from build123d import *

# Parameters (mm, degrees)
EXTRUDE_1_DEPTH        = 4
SKETCH_2_R             = 1.525
CUT_EXTRUDE_1_DEPTH    = 5
FILLET_1_R             = 3
SKETCH_3_R             = 1.8
CUT_EXTRUDE_5_DEPTH    = 5
CUT_EXTRUDE_3_DEPTH    = 5
FILLET_2_R             = 1.5
FILLET_2_OF_MIRROR_1_R = 1.5
SKETCH_5_R             = 9
CUT_EXTRUDE_4_DEPTH    = 5


with BuildPart() as part:
    # 草图1 → 凸台-拉伸1 (new body)
    with BuildSketch(Plane(origin=(0, 0, 0), x_dir=(1, 0, 0), z_dir=(0, 1, 0))):
        with BuildLine():
            Line((-20, 18), (-20, -18))
            Line((-20, -18), (20, -18))
            ThreePointArc((20, -18), (2, 0), (20, 18))
            Line((20, 18), (-20, 18))
        make_face()
        with BuildLine():
            ThreePointArc((20, 18), (2, 0), (20, -18))
            Line((20, -18), (20, 18))
        make_face()
        with BuildLine():
            Line((20, 18), (20, -18))
            ThreePointArc((20, -18), (32.727922061, -12.727922061), (38, 0))
            ThreePointArc((38, 0), (32.727922061, 12.727922061), (20, 18))
        make_face()
    extrude(amount=EXTRUDE_1_DEPTH)

    # 草图2 → 切除-拉伸1 (cut, through all)
    with BuildSketch(Plane(origin=(0, 4, 0), x_dir=(1, 0, 0), z_dir=(0, 1, 0))):
        with Locations((9.463257492, 8.439612392)):
            Circle(SKETCH_2_R)
        with Locations((7.422710017, -4.905280489)):
            Circle(SKETCH_2_R)
        with Locations((30.536742508, -8.439612392)):
            Circle(SKETCH_2_R)
        with Locations((17.959452524, -13.344892881)):
            Circle(SKETCH_2_R)
        with Locations((32.577289983, 4.905280489)):
            Circle(SKETCH_2_R)
        with Locations((22.040547476, 13.344892881)):
            Circle(SKETCH_2_R)
    extrude(amount=-CUT_EXTRUDE_1_DEPTH, mode=Mode.SUBTRACT)

    # 圆角1
    fillet_1_edges = [part.edges().sort_by_distance(p)[0] for p in [
        (-20, 2, 18),
        (-20, 2, -18),
    ]]
    fillet(fillet_1_edges, radius=FILLET_1_R)

    # 草图3 → 切除-拉伸5 (cut, through all)
    with BuildSketch(Plane(origin=(0, 4, 0), x_dir=(1, 0, 0), z_dir=(0, 1, 0))):
        with Locations((-17.5, -8.3)):
            Circle(SKETCH_3_R)
        with Locations((-17.5, 8.3)):
            Circle(SKETCH_3_R)
    extrude(amount=-CUT_EXTRUDE_5_DEPTH, mode=Mode.SUBTRACT)

    # 草图4 → 切除-拉伸3 (cut, through all)
    with BuildSketch(Plane(origin=(0, 4, 0), x_dir=(1, 0, 0), z_dir=(0, 1, 0))):
        Polygon((-11, 2), (-11, 13), (7, 13), align=None)
    cut_extrude_3 = extrude(amount=-CUT_EXTRUDE_3_DEPTH, mode=Mode.SUBTRACT)

    # 圆角2
    fillet_2_edges = [part.edges().sort_by_distance(p)[0] for p in [
        (-11, 2, -2),
        (-11, 2, -13),
        (7, 2, -13),
    ]]
    fillet(fillet_2_edges, radius=FILLET_2_R)

    # 镜向1: 切除-拉伸3 across plane
    add(cut_extrude_3.mirror(Plane.XY), mode=Mode.SUBTRACT)

    # 圆角2 of 镜向1
    fillet_2_of_mirror_1_edges = [part.edges().sort_by_distance(p)[0] for p in [
        (-11, 2, 2),
        (-11, 2, 13),
        (7, 2, 13),
    ]]
    fillet(fillet_2_of_mirror_1_edges, radius=FILLET_2_OF_MIRROR_1_R)

    # 草图5 → 切除-拉伸4 (cut, through all)
    with BuildSketch(Plane(origin=(0, 4, 0), x_dir=(1, 0, 0), z_dir=(0, 1, 0))):
        with Locations((20, 0)):
            Circle(SKETCH_5_R)
    extrude(amount=-CUT_EXTRUDE_4_DEPTH, mode=Mode.SUBTRACT)


solid = part.part
Build history of the part. All positions in model axes, mm. A direction names the side the tool comes from. Round coordinates to 2 decimals unless told otherwise and drop trailing zeros. Write each loop counter-clockwise with the first axis right and the second up, starting at its lowest first coordinate (ties: lowest second). Pieces come first, ordered by that corner, then holes. Notation, with made-up numbers: (23.25, 37) - (80.25, 37) arc R21 cw to (80.25, 61) - close; hole circle Ø10 at (17, -12.75). An arc over 180 degrees is marked (long way). Use CSV: the item, a comma, the result in double quotes.
(1) Mould opens along Z. For faces 1 (the cylindrical face through (-10.57, 1.97, 12.55)), 2 (the cylindrical face through (3.12, 1.97, -11.88)), 3 (the cylindrical face through (-19.1, 2.03, 17.14)), 4 (the cylindrical face through (-19.14, 2.03, -17.1)) say: pulls with the +Z half, pulls with the -Z half, needs draft (parallel to the pull), parting line crosses it, or undercut.
Response:
face 1,"undercut"
face 2,"undercut"
face 3,"pulls with the +Z half"
face 4,"pulls with the -Z half"
(2) 3-axis set-ups, long thin cutter, end or side, ignore diameter. For faces 5 (the flat face through (1, 2, 18)), 6 (the flat face through (-4, 2, 13)): which of +Z, -Z, +X, -X, +Y, -Y reach the whole face in a straight line?
Response:
face 5,"+Z, +X, -X, +Y, -Y"
face 6,"+Y, -Y"
(3) Band-saw the part on A-A (z = 2). Write the cut outline in (x, y), plus the area to 3 significant figures.
Response:
outline,"(-20, 0) - (11.23, 0) - (11.23, 4) - (-20, 4) - close; (28.77, 0) - (37.89, 0) - (37.89, 4) - (28.77, 4) - close"
area,"161 mm²"
(4) Pin check, flat tips, straight feed: P1, Ø1.2, axis at y = 2.5, z = -7, coming from the +X side; P2, Ø2, axis at y = 2.5, z = 7, coming from the +X side. Stop position of each tip, or through.
Response:
P1,"x = 36.82"
P2,"x = 36.97"
(5) Band-saw the part on C-C (x = 25.5). Write the cut outline in (y, z).
Response:
outline,"(0, -17.14) - (4, -17.14) - (4, -7.12) - (0, -7.12) - close; (0, 7.12) - (4, 7.12) - (4, 17.14) - (0, 17.14) - close"
(6) Band-saw the part on D-D (z = 7.5). Write the cut outline in (x, y).
Response:
outline,"(-20, 0) - (-19.11, 0) - (-19.11, 4) - (-20, 4) - close; (-15.89, 0) - (-11, 0) - (-11, 4) - (-15.89, 4) - close; (-2, 0) - (15.03, 0) - (15.03, 4) - (-2, 4) - close; (24.97, 0) - (29.34, 0) - (29.34, 4) - (24.97, 4) - close; (31.74, 0) - (36.36, 0) - (36.36, 4) - (31.74, 4) - close"
(7) Wall check: line 1 (Z direction, x = -0.5, y = 1.1); line 2 (Z direction, x = -16, y = 1.5); line 3 (X direction, y = 1.4, z = 6). Give the ranges that are in metal, low to high.
Response:
line 1,"-18 to -13, -8.42 to 8.42, 13 to 18"
line 2,"-18 to -9.29, -7.31 to 7.31, 9.29 to 18"
line 3,"-20 to -11, -4.45 to 6.36, 8.48 to 13.29, 26.71 to 36.97"
(8) Band-saw the part on B-B (x = -6). Write the cut outline in (y, z).
Response:
outline,"(0, -18) - (4, -18) - (4, -13) - (0, -13) - close; (0, -5.06) - (4, -5.06) - (4, 5.06) - (0, 5.06) - close; (0, 13) - (4, 13) - (4, 18) - (0, 18) - close"
